Input: part model. Units: mm. Frame: model coordinates. Face numbers are marked on the shaded views. Give positions to 0.01 mm unless a question says otherwise; leave off trailing zeros. Order: outer loops, then holes, each group sorted by start corner. A loop starts at its lowest first (then second) coordinate and runs counter-clockwise, first axis right, second up. Notation, with made-up numbers: (46.25, 86) - (59.25, 86) arc R12 cw to (59.25, 102) - close; hole circle Ø5 at (28, 35.25). An arc over 180 degrees is marked (long way). Use a Markdown table: item, result.
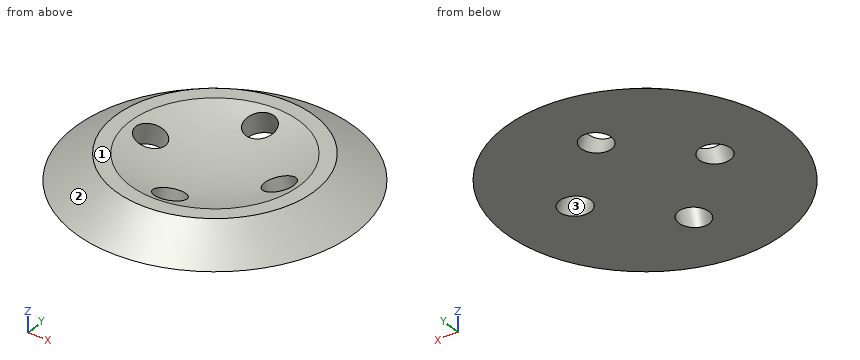
from build123d import *

# Parameters (mm, degrees)
PATTERN_CIRCULAR_1_COUNT = 4
MOVE_BODY_1_ANGLE        = 90


with BuildPart() as part:
    # 草图1 → 旋转1 (revolve)
    with BuildSketch(Plane(origin=(0, 0, 0), x_dir=(0, 0, -1), z_dir=(1, 0, 0)), mode=Mode.PRIVATE) as revolve_1_sk:
        with BuildLine():
            Line((0, 0), (0, -4.367835819))
            Line((0, -4.367835819), (60, -4.367835819))
            Line((60, -4.367835819), (42.679491924, 6.632164181))
            Line((42.679491924, 6.632164181), (36.32612495, 6.632164181))
            ThreePointArc((36.32612495, 6.632164181), (18.463294368, 1.671632263), (0, 0))
        make_face()
    revolve(revolve_1_sk.sketch.rotate(Axis((0, 23.869545483, 0), (0, -1, 0)), 180), axis=Axis((0, 23.869545483, 0), (0, -1, 0)))

    # 草图2 → 切除-旋转1 (revolve, cut)
    with BuildSketch(Plane.XY, mode=Mode.PRIVATE) as cut_revolve_1_sk:
        Polygon((23.11658969, 18.792484499), (29.364790714, 20.584127312), (39.564082896, -14.98503156), (33.315881872, -16.776674373), align=None)
    cut_revolve_1 = revolve(cut_revolve_1_sk.sketch.rotate(Axis((0, 99.409613277, 0), (0.2756373558169999, -0.9612616959383187, 0)), 180), axis=Axis((0, 99.409613277, 0), (0.2756373558169999, -0.9612616959383187, 0)), mode=Mode.SUBTRACT)

    # 阵列(圆周)1: 切除-旋转1 ×4 about axis
    pattern_circular_1_axis = Axis((0, 0, 0), (0, 1, 0))
    for i in range(1, PATTERN_CIRCULAR_1_COUNT):
        add(cut_revolve_1.rotate(pattern_circular_1_axis, i * 360 / PATTERN_CIRCULAR_1_COUNT), mode=Mode.SUBTRACT)


with BuildPart() as part_1:
    # Move Body 1: moved
    add(part.part.rotate(Axis((0, 1.132164181, 0), (1, 0, 0)), MOVE_BODY_1_ANGLE))


solid = part_1.part
1. Pin query (flat end, axial travel): pin 1 (5 mm diameter, centred on x = 20.5, y = 20.5, fed in from +Z); pin 2 (10 mm diameter, centred on x = 46, y = -32, fed in from +Z); pin 3 (4 mm diameter, centred on y = -16, z = -1, fed in from -X); pin 4 (10 mm diameter, centred on x = 46.5, y = 42.5, fed in from -Z). Return the tip coordinate at first contact, or that it passes through.
Response:
| item | result |
|---|---|
| pin 1 | stops at z = 3.56 |
| pin 2 | stops at z = -0.22 |
| pin 3 | stops at x = -53.44 |
| pin 4 | stops at z = -5.5 |
2. Mould query, pull axis Y, two halves, no side actions, for the marked faces 1, 2 and 3. Classes: pulls with the +Y half, pulls with the -Y half, needs draft (parallel to the pull), parting line crosses it, or undercut.
Response:
| item | result |
|---|---|
| face 1 | needs draft |
| face 2 | parting line crosses it |
| face 3 | undercut |
3. Material intervals for line 1 along X through (y, z) = (2, -3); line 2 along Y through (x, z) = (-1, -4.5); line 3 along X through (y, z) = (34.5, -2), sorted ascending.
Response:
| item | result |
|---|---|
| line 1 | x = -56.06 to -35.74, -22.34 to 22.34, 35.74 to 56.06 |
| line 2 | y = -57.28 to -35.02, -21.66 to 23.92, 37.28 to 59.55 |
| line 3 | x = -43.08 to -4.75, 4.75 to 43.08 |
4. Section query A-A (x = 0). Return loops of the section in (y, z), then the cut area to 3 significant figures.
Response:
| item | result |
|---|---|
| outline | (-58.87, -5.5) - (-35.39, -5.5) - (-32.51, 4.53) arc R102.8 cw to (-35.19, 5.5) - (-41.55, 5.5) - close; (-21.86, -5.5) - (24.13, -5.5) - (22.25, 1.06) arc R102.8 cw to (-19.98, 1.06) - close; (34.78, 4.53) - (37.65, -5.5) - (61.13, -5.5) - (43.81, 5.5) - (37.46, 5.5) arc R102.8 cw to start |
| area | 585 mm^2 |
